from build123d import *

# Parameters (mm, degrees)
SKETCH_1_W          = 49
SKETCH_1_H          = 1.2
EXTRUDE_1_DEPTH     = 22
CUT_EXTRUDE_1_REACH = 55.726
SKETCH_2_R          = 2
SKETCH_3_W          = 2
SKETCH_3_H          = 25
EXTRUDE_2_DEPTH     = 25
CUT_EXTRUDE_2_REACH = 61.762
SKETCH_4_R          = 7.25
SKETCH_5_R          = 8
SKETCH_5_R_2        = 7.25
EXTRUDE_3_DEPTH     = 3
EXTRUDE_START       = -1
SKETCH_6_R          = 8
SKETCH_6_R_2        = 6.5
EXTRUDE_4_DEPTH     = 1
EXTRUDE_5_REACH     = 60.107
SKETCH_7_W          = 2
SKETCH_7_H          = 6.3
FILLET_1_R          = 10
EXTRUDE_6_DEPTH     = 1.2


with BuildPart() as part:
    # 草图1 → 凸台-拉伸1 (new body)
    with BuildSketch(Plane(origin=(0, 0, 0), x_dir=(0, 0, -1), z_dir=(1, 0, 0))):
        with Locations((24.5, 0.6)):
            Rectangle(SKETCH_1_W, SKETCH_1_H)
    extrude(amount=EXTRUDE_1_DEPTH)

    # 草图2 → 切除-拉伸1 (cut, up to next)
    with BuildSketch(Plane(origin=(0, 1.2, 0), x_dir=(1, 0, 0), z_dir=(0, 1, 0)), mode=Mode.PRIVATE) as cut_extrude_1_sk1:
        with Locations(Location((16, 19, 0), (0, 0, 270))):
            Circle(SKETCH_2_R)
    cut_extrude_1_tool1 = extrude(cut_extrude_1_sk1.sketch, amount=-CUT_EXTRUDE_1_REACH, mode=Mode.PRIVATE) & part.part
    # 草图2 → 切除-拉伸1 (cut, up to next)
    with BuildSketch(Plane(origin=(0, 1.2, 0), x_dir=(1, 0, 0), z_dir=(0, 1, 0)), mode=Mode.PRIVATE) as cut_extrude_1_sk2:
        with Locations(Location((4, 19, 0), (0, 0, 270))):
            Circle(SKETCH_2_R)
    cut_extrude_1_tool2 = extrude(cut_extrude_1_sk2.sketch, amount=-CUT_EXTRUDE_1_REACH, mode=Mode.PRIVATE) & part.part
    # 草图2 → 切除-拉伸1 (cut, up to next)
    with BuildSketch(Plane(origin=(0, 1.2, 0), x_dir=(1, 0, 0), z_dir=(0, 1, 0)), mode=Mode.PRIVATE) as cut_extrude_1_sk3:
        with Locations(Location((4, 4, 0), (0, 0, 270))):
            Circle(SKETCH_2_R)
    cut_extrude_1_tool3 = extrude(cut_extrude_1_sk3.sketch, amount=-CUT_EXTRUDE_1_REACH, mode=Mode.PRIVATE) & part.part
    # 草图2 → 切除-拉伸1 (cut, up to next)
    with BuildSketch(Plane(origin=(0, 1.2, 0), x_dir=(1, 0, 0), z_dir=(0, 1, 0)), mode=Mode.PRIVATE) as cut_extrude_1_sk4:
        with Locations(Location((16, 4, 0), (0, 0, 270))):
            Circle(SKETCH_2_R)
    cut_extrude_1_tool4 = extrude(cut_extrude_1_sk4.sketch, amount=-CUT_EXTRUDE_1_REACH, mode=Mode.PRIVATE) & part.part
    add(cut_extrude_1_tool1.solids().sort_by_distance((16, 1.2, -19))[0], mode=Mode.SUBTRACT)
    add(cut_extrude_1_tool2.solids().sort_by_distance((4, 1.2, -19))[0], mode=Mode.SUBTRACT)
    add(cut_extrude_1_tool3.solids().sort_by_distance((4, 1.2, -4))[0], mode=Mode.SUBTRACT)
    add(cut_extrude_1_tool4.solids().sort_by_distance((16, 1.2, -4))[0], mode=Mode.SUBTRACT)

    # 草图3 → 凸台-拉伸2 (add)
    with BuildSketch(Plane(origin=(0, 1.2, 0), x_dir=(1, 0, 0), z_dir=(0, 1, 0))):
        with Locations((21, 36.5)):
            Rectangle(SKETCH_3_W, SKETCH_3_H)
    extrude(amount=EXTRUDE_2_DEPTH)

    # 草图4 → 切除-拉伸2 (cut, up to next)
    with BuildSketch(Plane(origin=(22, 0, 0), x_dir=(0, 0, -1), z_dir=(1, 0, 0)), mode=Mode.PRIVATE) as cut_extrude_2_sk1:
        with Locations((37.15, 14)):
            Circle(SKETCH_4_R)
    cut_extrude_2_tool1 = extrude(cut_extrude_2_sk1.sketch, amount=-CUT_EXTRUDE_2_REACH, mode=Mode.PRIVATE) & part.part
    add(cut_extrude_2_tool1.solids().sort_by_distance((22, 14, -37.15))[0], mode=Mode.SUBTRACT)

    # 草图5 → 凸台-拉伸3 (add)
    with BuildSketch(Plane.ZY.offset(-20)):
        with Locations(Location((-37.15, 14, 0), (0, 0, 180))):
            Circle(SKETCH_5_R)
        with Locations(Location((-37.15, 14, 0), (0, 0, 180))):
            Circle(SKETCH_5_R_2, mode=Mode.SUBTRACT)
    extrude(amount=EXTRUDE_3_DEPTH)

    # 草图6 → 凸台-拉伸4 (add)
    with BuildSketch(Plane.ZY.offset(-17).offset(EXTRUDE_START)):
        with Locations(Location((-37.15, 14, 0), (0, 0, 180))):
            Circle(SKETCH_6_R)
        with Locations((-37.15, 14)):
            Circle(SKETCH_6_R_2, mode=Mode.SUBTRACT)
    extrude(amount=EXTRUDE_4_DEPTH)

    # 草图7 → 凸台-拉伸5 (add, up to next)
    with BuildSketch(Plane.ZY.offset(-17), mode=Mode.PRIVATE) as extrude_5_sk1:
        with Locations((-37.15, 4.35)):
            Rectangle(SKETCH_7_W, SKETCH_7_H)
    extrude_5_tool1 = extrude(extrude_5_sk1.sketch, amount=-EXTRUDE_5_REACH, mode=Mode.PRIVATE) - part.part
    add(extrude_5_tool1.solids().sort_by_distance((17, 4.35, -37.15))[0])

    # 圆角1
    fillet_1_edges = [part.edges().sort_by_distance(p)[0] for p in [
        (21, 26.2, -24),
        (21, 26.2, -49),
    ]]
    fillet(fillet_1_edges, radius=FILLET_1_R)

    # 草图8 → 凸台-拉伸6 (add)
    with BuildSketch(Plane(origin=(22, 0, 0), x_dir=(0, 0, -1), z_dir=(1, 0, 0))):
        Polygon((0, 1.2), (24, 16.2), (24, 1.2), align=None)
    extrude(amount=-EXTRUDE_6_DEPTH)


solid = part.part
Verification items for the finished model (mm, model axes). A direction names the side the tool comes from. Coordinates: 2 decimals unless noted, no trailing zeros. Loops run counter-clockwise (first coordinate to the right, second up) from the corner with the lowest first, then second, coordinate; pieces in that order, holes last. Notation, with made-up numbers: (3.25, 85.5) -> (15.25, 85.5) arc R22 ccw to (15.25, 124.5) -> close; hole circle Ø9 at (85.25, -14.75). An arc over 180 degrees is marked (long way). Answer as a JSON object with one key per item and string values. Group by question number.
Item 1: Sectioned sample at C-C on z = -37.15. Record the boundary of the cut face in (x, y), plus the area to 3 significant figures.
Item 2: Tool access check on faces 1 (the flat face through (18, 4, -38.15)), 2 (the cylindrical face through (19, 22, -37)), 3 (the cylindrical face through (20.028, 11.822, -44.065)), 4 (the flat face through (20.8, 5, -18)), 5 (the flat face through (18, 4, -36.15)). Record the directions out of +Z, -Z, +X, -X, +Y, -Y that give a thin tool (end or side, any length) a straight path to the whole face; none if there is none.
Item 3: Depth check by flat-ended pin: pin 1 (3 mm diameter, centred on y = 8.5, z = -11.5, fed in from +X); pin 2 (1.5 mm diameter, centred on x = 13, z = -44, fed in from +Y); pin 3 (3.5 mm diameter, centred on x = 19, y = 3.5, fed in from +Z); pin 4 (10 mm diameter, centred on y = 10, z = -22, fed in from -X). Enter the tip coordinate at first touch or a pass-through.
Item 4: Sectioned sample at D-D on x = 18.5. Record the boundary of the cut face in (y, z), plus the area to 3 significant figures.
Item 5: Scan lines: probe 1 along X at (y, z) = (0.9, -4); probe 2 along Y at (x, z) = (20.85, -37.15); probe 3 along Y at (x, z) = (17.25, -38.5). Record each from-to range of solid material in increasing order.
Item 6: Mould release check, pull along Z, two halves, no side actions. Record for faces 6 (the flat face through (11, 0, -24)), 7 (the cylindrical face through (21.01, 23.35, -45.99)), 8 (the cylindrical face through (18, 1, -19)), 9 (the flat face through (18, 8, -34)): +Z half, -Z half, draft (parallel to the pull), parting line (faces both ways), or undercut.
Item 7: Sectioned sample at A-A on z = -4. Record the boundary of the cut face in (x, y).
Item 8: Sectioned sample at B-B on x = 16. Record the boundary of the cut face in (y, z).
Evaluation:
{
 "1": {"outline": "(0, 0) -> (22, 0) -> (22, 6.75) -> (18, 6.75) -> (18, 7.5) -> (17, 7.5) -> (17, 1.2) -> (0, 1.2) -> close; (17, 20.5) -> (18, 20.5) -> (18, 21.25) -> (22, 21.25) -> (22, 26.2) -> (20, 26.2) -> (20, 22) -> (17, 22) -> close", "area": "67.8 mm²"},
 "2": {"face 1": "-Z, -X", "face 2": "-X", "face 3": "+X", "face 4": "+Z, -X, +Y", "face 5": "+Z, -X"},
 "3": {"pin 1": "stops at x = 22", "pin 2": "stops at y = 1.2", "pin 3": "stops at z = -24", "pin 4": "stops at x = 20"},
 "4": {"outline": "(0, -49) -> (1.2, -49) -> (1.2, -38.15) -> (6.06, -38.15) arc R8 ccw (long way) to (6.06, -36.15) -> (1.2, -36.15) -> (1.2, 0) -> (0, 0) -> close; hole circle Ø14.5 at (14, -37.15)", "area": "104 mm²"},
 "5": {"probe 1": "x = 0 to 2, 6 to 14, 18 to 22", "probe 2": "y = 0 to 6.75, 21.25 to 26.2", "probe 3": "y = 0 to 1.2, 6.11 to 7.64, 20.36 to 21.89"},
 "6": {"face 6": "draft", "face 7": "-Z half", "face 8": "undercut", "face 9": "undercut"},
 "7": {"outline": "(0, 0) -> (2, 0) -> (2, 1.2) -> (0, 1.2) -> close; (6, 0) -> (14, 0) -> (14, 1.2) -> (6, 1.2) -> close; (18, 0) -> (22, 0) -> (22, 3.7) -> (20.8, 3.7) -> (20.8, 1.2) -> (18, 1.2) -> close"},
 "8": {"outline": "(0, -49) -> (1.2, -49) -> (1.2, -21) -> (0, -21) -> close; (0, -17) -> (1.2, -17) -> (1.2, -6) -> (0, -6) -> close; (0, -2) -> (1.2, -2) -> (1.2, 0) -> (0, 0) -> close"}
}
